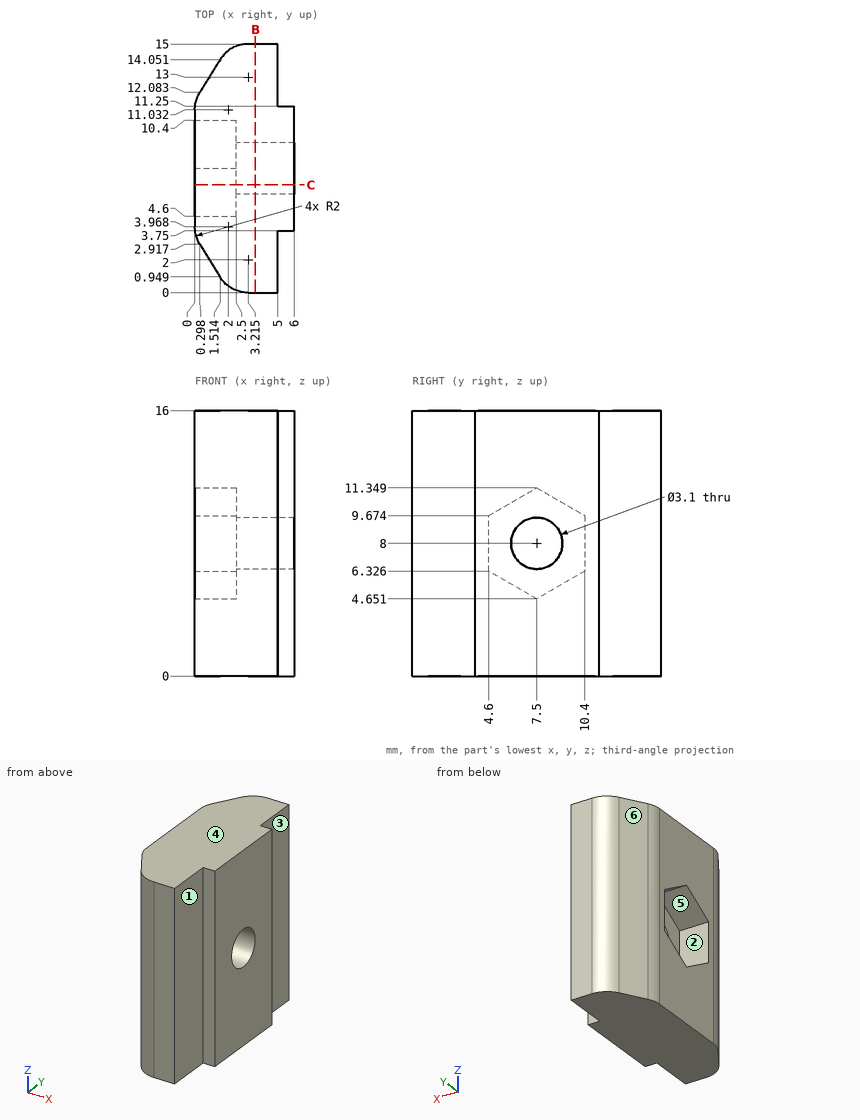
Part print with two shaded views. Sizes in mm from the minimum x, y, z corner. A direction names the side the tool comes from. Round coordinates to 2 decimals unless told otherwise and drop trailing zeros. Order: outer loops, then holes, each group sorted by start corner. A loop starts at its lowest first (then second) coordinate and runs counter-clockwise, first axis right, second up. Notation, with made-up numbers: (10, -16) - (15, -16) arc R20 cw to (15, -6) - close; hole circle Ø7 at (64.5, 68.25). An arc over 180 degrees is marked (long way). Return JSON: item names as keys, results as strings.
(1) Pin check, flat tips, straight feed: pin 1 Ø0.8 at (x, z) = (1, 8.5) entering from +Y (1 decimal); pin 2 Ø1.9 at (y, z) = (2, 10.5) entering from +X; pin 3 Ø0.8 at (x, z) = (1, 7.5) entering from -Y (1 decimal). Stop position of each tip, or through.
Answer key:
{"pin 1": "stops at y = 13.9", "pin 2": "stops at x = 5", "pin 3": "stops at y = 1.1"}
(2) Wall check: probe 1 along Y at (x, z) = (5.35, 8); probe 2 along Z at (x, y) = (4.25, 7.5); probe 3 along Y at (x, z) = (4.9, 8). Give the ranges that are in metal, low to high. Write a range as from..to.
Answer key:
{"probe 1": "y = 3.75..5.95, 9.05..11.25", "probe 2": "z = 0..6.45, 9.55..16", "probe 3": "y = 0..5.95, 9.05..15"}
(3) Pull direction Z, two halves, no side cores. Call the marked faces 4, 5 and 6: +Z half, -Z half, draft (parallel to the pull), parting line (faces both ways), or undercut.
Answer key:
{"face 4": "+Z half", "face 5": "undercut", "face 6": "draft"}
(4) Cut at B-B (x = 3.65). Give the cut face in (y, z).
Answer key:
{"outline": "(0, 0) - (15, 0) - (15, 16) - (0, 16) - close; hole circle Ø3.1 at (7.5, 8)"}
(5) Cut at C-C (y = 6.5). Give the cut face in (x, z) (1 decimal).
Answer key:
{"outline": "(0, 0) - (6, 0) - (6, 6.8) - (2.5, 6.8) - (2.5, 5.2) - (0, 5.2) - close; (0, 10.8) - (2.5, 10.8) - (2.5, 9.2) - (6, 9.2) - (6, 16) - (0, 16) - close"}
(6) Tool access for the marked faces 1, 2 and 3: list every direction of +Z, -Z, +X, -X, +Y, -Y with a clear straight run to the whole face (end or side of a thin tool).
Answer key:
{"face 1": "+Z, -Z, +X, -Y", "face 2": "-X", "face 3": "+Z, -Z, +X, +Y"}
